from build123d import *

# Parameters (mm, degrees)
F1_DEPTH = 4
F2_DEPTH = 1.5
F3_SIZE  = 2


with BuildPart() as f1:
    # F0 (on Front) → F1 (new body)
    with BuildSketch(Plane.XZ):
        with BuildLine():
            ThreePointArc((-12.41, 1.4972975656), (-12.1967325212, 2.7367345149), (-11.86, 3.9484680574))
            ThreePointArc((-11.86, 3.9484680574), (-12.1789643551, 3.9870962008), (-12.5, 4))
            ThreePointArc((-12.5, 4), (-16.5, 0), (-12.5, -4))
            ThreePointArc((-12.5, -4), (-12.1789643551, -3.9870962008), (-11.86, -3.9484680574))
            ThreePointArc((-11.86, -3.9484680574), (-12.1967325212, -2.7367345149), (-12.41, -1.4972975656))
            ThreePointArc((-12.41, -1.4972975656), (-14, 0), (-12.41, 1.4972975656))
        make_face()
        with BuildLine():
            Line((-11, 0), (-8.5, 0))
            ThreePointArc((-8.5, 0), (-9.4536907577, 2.5922962794), (-11.86, 3.9484680574))
            ThreePointArc((-11.86, 3.9484680574), (-12.1967325212, 2.7367345149), (-12.41, 1.4972975656))
            ThreePointArc((-12.41, 1.4972975656), (-11.4079835166, 1.0283481901), (-11, 0))
        make_face()
        with BuildLine():
            ThreePointArc((-11.86, -3.9484680574), (-9.4536907577, -2.5922962794), (-8.5, 0))
            Line((-8.5, 0), (-11, 0))
            ThreePointArc((-11, 0), (-11.4079835166, -1.0283481901), (-12.41, -1.4972975656))
            ThreePointArc((-12.41, -1.4972975656), (-12.1967325212, -2.7367345149), (-11.86, -3.9484680574))
        make_face()
        with BuildLine():
            ThreePointArc((11.8427192823, -4), (11.85138765, -3.9742434211), (11.86, -3.9484680574))
            ThreePointArc((11.86, -3.9484680574), (9.4536907577, -2.5922962794), (8.5, 0))
            Line((8.5, 0), (-8.5, 0))
            ThreePointArc((-8.5, 0), (-9.4536907577, -2.5922962794), (-11.86, -3.9484680574))
            ThreePointArc((-11.86, -3.9484680574), (-11.85138765, -3.9742434211), (-11.8427192823, -4))
            Line((-11.8427192823, -4), (11.8427192823, -4))
        make_face()
        with BuildLine():
            ThreePointArc((8.5, 0), (9.4536907577, 2.5922962794), (11.86, 3.9484680574))
            ThreePointArc((11.86, 3.9484680574), (11.85138765, 3.9742434211), (11.8427192823, 4))
            Line((11.8427192823, 4), (-11.8427192823, 4))
            ThreePointArc((-11.8427192823, 4), (-11.85138765, 3.9742434211), (-11.86, 3.9484680574))
            ThreePointArc((-11.86, 3.9484680574), (-9.4536907577, 2.5922962794), (-8.5, 0))
            Line((-8.5, 0), (8.5, 0))
        make_face()
        with BuildLine():
            ThreePointArc((11, 0), (11.4079835166, 1.0283481901), (12.41, 1.4972975656))
            ThreePointArc((12.41, 1.4972975656), (12.1967325212, 2.7367345149), (11.86, 3.9484680574))
            ThreePointArc((11.86, 3.9484680574), (9.4536907577, 2.5922962794), (8.5, 0))
            Line((8.5, 0), (11, 0))
        make_face()
        with BuildLine():
            ThreePointArc((11.86, -3.9484680574), (12.1967325212, -2.7367345149), (12.41, -1.4972975656))
            ThreePointArc((12.41, -1.4972975656), (11.4079835166, -1.0283481901), (11, 0))
            Line((11, 0), (8.5, 0))
            ThreePointArc((8.5, 0), (9.4536907577, -2.5922962794), (11.86, -3.9484680574))
        make_face()
        with BuildLine():
            ThreePointArc((11.86, 3.9484680574), (12.1967325212, 2.7367345149), (12.41, 1.4972975656))
            ThreePointArc((12.41, 1.4972975656), (13.5283481901, 1.0920164834), (14, 0))
            ThreePointArc((14, 0), (13.5283481901, -1.0920164834), (12.41, -1.4972975656))
            ThreePointArc((12.41, -1.4972975656), (12.1967325212, -2.7367345149), (11.86, -3.9484680574))
            ThreePointArc((11.86, -3.9484680574), (12.1789643551, -3.9870962008), (12.5, -4))
            ThreePointArc((12.5, -4), (15.3284271247, -2.8284271247), (16.5, 0))
            ThreePointArc((16.5, 0), (15.3284271247, 2.8284271247), (12.5, 4))
            ThreePointArc((12.5, 4), (12.1789643551, 3.9870962008), (11.86, 3.9484680574))
        make_face()
    extrude(amount=F1_DEPTH)

    # F0 (on Front) → F2 (cut)
    with BuildSketch(Plane.XZ):
        with BuildLine():
            ThreePointArc((11.8427192823, -4), (11.85138765, -3.9742434211), (11.86, -3.9484680574))
            ThreePointArc((11.86, -3.9484680574), (9.4536907577, -2.5922962794), (8.5, 0))
            Line((8.5, 0), (-8.5, 0))
            ThreePointArc((-8.5, 0), (-9.4536907577, -2.5922962794), (-11.86, -3.9484680574))
            ThreePointArc((-11.86, -3.9484680574), (-11.85138765, -3.9742434211), (-11.8427192823, -4))
            Line((-11.8427192823, -4), (11.8427192823, -4))
        make_face()
        with BuildLine():
            ThreePointArc((8.5, 0), (9.4536907577, 2.5922962794), (11.86, 3.9484680574))
            ThreePointArc((11.86, 3.9484680574), (11.85138765, 3.9742434211), (11.8427192823, 4))
            Line((11.8427192823, 4), (-11.8427192823, 4))
            ThreePointArc((-11.8427192823, 4), (-11.85138765, 3.9742434211), (-11.86, 3.9484680574))
            ThreePointArc((-11.86, 3.9484680574), (-9.4536907577, 2.5922962794), (-8.5, 0))
            Line((-8.5, 0), (8.5, 0))
        make_face()
    extrude(amount=F2_DEPTH, mode=Mode.SUBTRACT)

    # F3
    f3_edges = [f1.edges().sort_by_distance(p)[0] for p in [
        (-14, -4, 0),
        (12.59, -4, -1.497298),
    ]]
    chamfer(f3_edges, length=F3_SIZE)


solid = f1.part
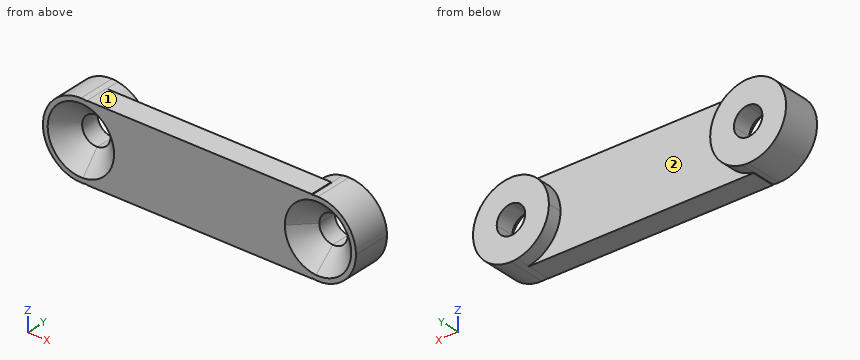
Can you work these out from the model? Positions are in its coordinate system, mm. Face numbers are marked on the shaded views. Round coordinates to 2 decimals unless told otherwise and drop trailing zeros. Order: outer loops, then holes, each group sorted by start corner. A loop starts at its lowest first (then second) coordinate and runs counter-clockwise, first axis right, second up. Notation, with made-up numbers: (-37.5, 72.5) -> (-20.5, 72.5) arc R8 ccw to (-20.5, 82.5) -> close; hole circle Ø9 at (-29.75, 68). An arc over 180 degrees is marked (long way). Write each question's results on one line, items separated by ' | '. Start each with the question number.
Item 1: If we section it at B-B, the plane y = -2.5: Write out the boundary of the cut face in (x, z), then the cut area to 3 significant figures.
Item 2: If we section it at A-A, the plane y = -1.05: Write out the boundary of the cut face in (x, z).
Item 3: Will these pins go through, and if not, where does the flat tip stop? pin 1 (4 mm diameter, centred on x = -3.5, z = -1.5, fed in from +Y); pin 2 (2 mm diameter, centred on x = -11.5, z = -2, fed in from +Y).
Item 4: If we section it at D-D, the plane z = -0.5: State how many separate pieces and enclosed holes the cut face has, then the cut area to 3 significant figures.
Item 5: If we section it at C-C, the plane x = -7.5: Write out the boundary of the cut face in (y, z).
Item 6: Please list where these lines run through material, in increasing order: L1, parallel to X at y = -3.7, z = 0.75; L2, parallel to Z at x = -12.5, y = -0.6; L3, parallel to Y at x = -7, z = -0.5.
Item 7: Thinking about a two-plate mould opening in X: for the marked faces 1 and 2, which applies, +X half, -X half, draft (parallel to the pull), parting line (faces both ways), or undercut?
Results:
1) outline: (-11.86, -3.95) arc R12.5 ccw to (-11.84, -4) -> (11.84, -4) arc R12.5 ccw to (11.86, -3.95) arc R4 ccw (long way) to (11.86, 3.95) arc R12.5 ccw to (11.84, 4) -> (-11.84, 4) arc R12.5 ccw to (-11.86, 3.95) arc R4 ccw (long way) to start; hole circle Ø4 at (-12.5, 0); hole circle Ø4 at (12.5, 0) | area: 225 mm2
2) outline: circle Ø8 at (-12.5, 0); circle Ø8 at (12.5, 0); hole circle Ø3 at (-12.5, 0); hole circle Ø3 at (12.5, 0)
3) pin 1: stops at y = -1.5 | pin 2: stops at y = 0
4) separate pieces: 3 | enclosed holes: 0 | area: 75.3 mm2
5) outline: (-4, -4) -> (-1.5, -4) -> (-1.5, 4) -> (-4, 4) -> close
6) L1: x = -16.43 to -15.61, -9.39 to 9.39, 15.61 to 16.43 | L2: z = -4 to -1.5, 1.5 to 4 | L3: y = -4 to -1.5
7) face 1: draft | face 2: undercut
